Here's how the part is built. I have some questions about the finished solid (model axes, mm). A direction names the side the tool comes from. Give positions to 0.01 mm unless a question says otherwise; leave off trailing zeros. Write each loop counter-clockwise with the first axis right and the second up, starting at its lowest first coordinate (ties: lowest second). Pieces come first, ordered by that corner, then holes. Notation, with made-up numbers: (0.25, 22) - (26.25, 22) arc R15 ccw to (26.25, 41) - close; hole circle Ø6 at (7.5, -18). An arc over 180 degrees is marked (long way). Use a Markdown table: item, result.
```python
from build123d import *

# Parameters (mm, degrees)
F0_W     = 100
F0_H     = 20
F1_DEPTH = 6
F2_R     = 5
F4_DEPTH = 6
F5_R     = 5
F7_DEPTH = 37


with BuildPart() as f1:
    # F0 (on Front) → F1 (new body)
    with BuildSketch(Plane.XZ):
        Rectangle(F0_W, F0_H)
    extrude(amount=F1_DEPTH)

    # F2
    f2_edges = [f1.edges().sort_by_distance(p)[0] for p in [
        (50, -3, 10),
        (50, -3, -10),
    ]]
    fillet(f2_edges, radius=F2_R)

    # F3 (on face) → F4 (join)
    with BuildSketch(Plane.XZ.offset(6)):
        with BuildLine():
            Line((45, 10), (0, 10))
            Line((0, 10), (0, -10))
            Line((0, -10), (45, -10))
            ThreePointArc((45, -10), (48.5355339059, -8.5355339059), (50, -5))
            Line((50, -5), (50, 5))
            ThreePointArc((50, 5), (48.5355339059, 8.5355339059), (45, 10))
        make_face()
    extrude(amount=F4_DEPTH)

    # F5
    f5_edges = [f1.edges().sort_by_distance(p)[0] for p in [
        (22.5, -12, 10),
    ]]
    fillet(f5_edges, radius=F5_R)

    # F6 (on Front) → F7 (cut)
    with BuildSketch(Plane.XZ):
        with BuildLine():
            ThreePointArc((15, 11.9532615303), (12.4128794991, 15.6125178063), (11.5, 20))
            ThreePointArc((11.5, 20), (12.4128794991, 24.3874821937), (15, 28.0467384697))
            ThreePointArc((15, 28.0467384697), (-3.5, 20), (15, 11.9532615303))
        make_face()
        with BuildLine():
            ThreePointArc((48.5, 20), (41.8874821937, 30.0871205009), (30, 28.0467384697))
            ThreePointArc((30, 28.0467384697), (32.5871205009, 24.3874821937), (33.5, 20))
            ThreePointArc((33.5, 20), (32.5871205009, 15.6125178063), (30, 11.9532615303))
            ThreePointArc((30, 11.9532615303), (41.8874821937, 9.9128794991), (48.5, 20))
        make_face()
        with BuildLine():
            Line((26.5, 20), (18.5, 20))
            ThreePointArc((18.5, 20), (17.5871205009, 15.6125178063), (15, 11.9532615303))
            ThreePointArc((15, 11.9532615303), (22.5, 9), (30, 11.9532615303))
            ThreePointArc((30, 11.9532615303), (27.4128794991, 15.6125178063), (26.5, 20))
        make_face()
        with BuildLine():
            ThreePointArc((15, -28.0467384697), (11.5, -20), (15, -11.9532615303))
            ThreePointArc((15, -11.9532615303), (-3.5, -20), (15, -28.0467384697))
        make_face()
        with BuildLine():
            ThreePointArc((15, -11.9532615303), (17.5871205009, -15.6125178063), (18.5, -20))
            ThreePointArc((18.5, -20), (17.5871205009, -24.3874821937), (15, -28.0467384697))
            ThreePointArc((15, -28.0467384697), (22.5, -31), (30, -28.0467384697))
            ThreePointArc((30, -28.0467384697), (26.5, -20), (30, -11.9532615303))
            ThreePointArc((30, -11.9532615303), (22.5, -9), (15, -11.9532615303))
        make_face()
        with BuildLine():
            ThreePointArc((48.5, -20), (41.8874821937, -9.9128794991), (30, -11.9532615303))
            ThreePointArc((30, -11.9532615303), (32.5871205009, -15.6125178063), (33.5, -20))
            ThreePointArc((33.5, -20), (32.5871205009, -24.3874821937), (30, -28.0467384697))
            ThreePointArc((30, -28.0467384697), (41.8874821937, -30.0871205009), (48.5, -20))
        make_face()
    extrude(amount=F7_DEPTH, mode=Mode.SUBTRACT)


solid = f1.part
```
Item 1: Thinking about a two-plate mould opening in X: for faces 3 (the cylindrical face through (7.4, -4.9, 9)), 4 (the flat face through (-24, -3, -10)), 5 (the cylindrical face through (49, -10, 0)), which applies, +X half, -X half, draft (parallel to the pull), parting line (faces both ways), or undercut?
Values:
| item | result |
|---|---|
| face 3 | undercut |
| face 4 | draft |
| face 5 | +X half |
Item 2: If we section it at D-D, the plane y = -8.5: Write out the boundary of the cut face in (x, z), plus the area to 3 significant figures.
Values:
| item | result |
|---|---|
| outline | (0, -9.77) - (3.46, -9.77) arc R11 cw to (11.54, -9.77) - (18.46, -9.77) arc R11 cw to (26.54, -9.77) - (33.46, -9.77) arc R11 cw to (41.54, -9.77) - (45, -9.77) arc R4.77 ccw to (49.77, -5) - (49.77, 5) arc R4.77 ccw to (45, 9.77) - (41.54, 9.77) arc R11 cw to (33.46, 9.77) - (26.54, 9.77) arc R11 cw to (18.46, 9.77) - (11.54, 9.77) arc R11 cw to (3.46, 9.77) - (0, 9.77) - close |
| area | 938 mm2 |
Item 3: If we section it at B-B, the plane x = 2: Write out the boundary of the cut face in (y, z).
Values:
| item | result |
|---|---|
| outline | (-12, -5) arc R5 ccw to (-7, -10) - (0, -10) - (0, 10) - (-7, 10) arc R5 ccw to (-12, 5) - close |
Item 4: If we section it at A-A, the plane z = -3.75: Write out the boundary of the cut face in (x, y).
Values:
| item | result |
|---|---|
| outline | (-50, -6) - (0, -6) - (0, -12) - (45, -12) arc R5 ccw to (50, -7) - (50, 0) - (-50, 0) - close |
Item 5: Will these pins go through, and if not, where does the flat tip stop? pin 1 Ø4 at (x, y) = (27, -10) entering from -Z; pin 2 Ø1 at (x, z) = (-9.5, -4) entering from -Y; pin 3 Ø2 at (y, z) = (-9, -4) entering from -X.
Values:
| item | result |
|---|---|
| pin 1 | stops at z = -9.9 |
| pin 2 | stops at y = -6 |
| pin 3 | stops at x = 0 |
Item 6: For faces 1 (the flat face through (-25, -6, 0)), 2 (the cylindrical face through (22.82, -10.5, -8.57)), which set-ups out of +Z, -Z, +X, -X, +Y, -Y let a thin tool reach every point of the face, with its end or its side?
Values:
| item | result |
|---|---|
| face 1 | +Z, -Z, -X, -Y |
| face 2 | -Z, +X, -X, -Y |
Item 7: If we section it at C-C, the plane y = -4.75: Write out the boundary of the cut face in (x, z).
Values:
| item | result |
|---|---|
| outline | (-50, -10) - (2.92, -10) arc R11 cw to (12.08, -10) - (17.92, -10) arc R11 cw to (27.08, -10) - (32.92, -10) arc R11 cw to (42.08, -10) - (45, -10) arc R5 ccw to (50, -5) - (50, 5) arc R5 ccw to (45, 10) - (42.08, 10) arc R11 cw to (32.92, 10) - (27.08, 10) arc R11 cw to (17.92, 10) - (12.08, 10) arc R11 cw to (2.92, 10) - (-50, 10) - close |
Item 8: I need wall thicknesses on line 1 along Y through (x, z) = (-14.5, 4.75); line 2 along Z through (x, y) = (38, -10); line 3 along X through (y, z) = (-6.5, 3). Which ranges of each line are inside material? Lowest first, please. Write a range as [from, to].
Values:
| item | result |
|---|---|
| line 1 | y = [-6, 0] |
| line 2 | z = [-9, 9] |
| line 3 | x = [0, 50] |
